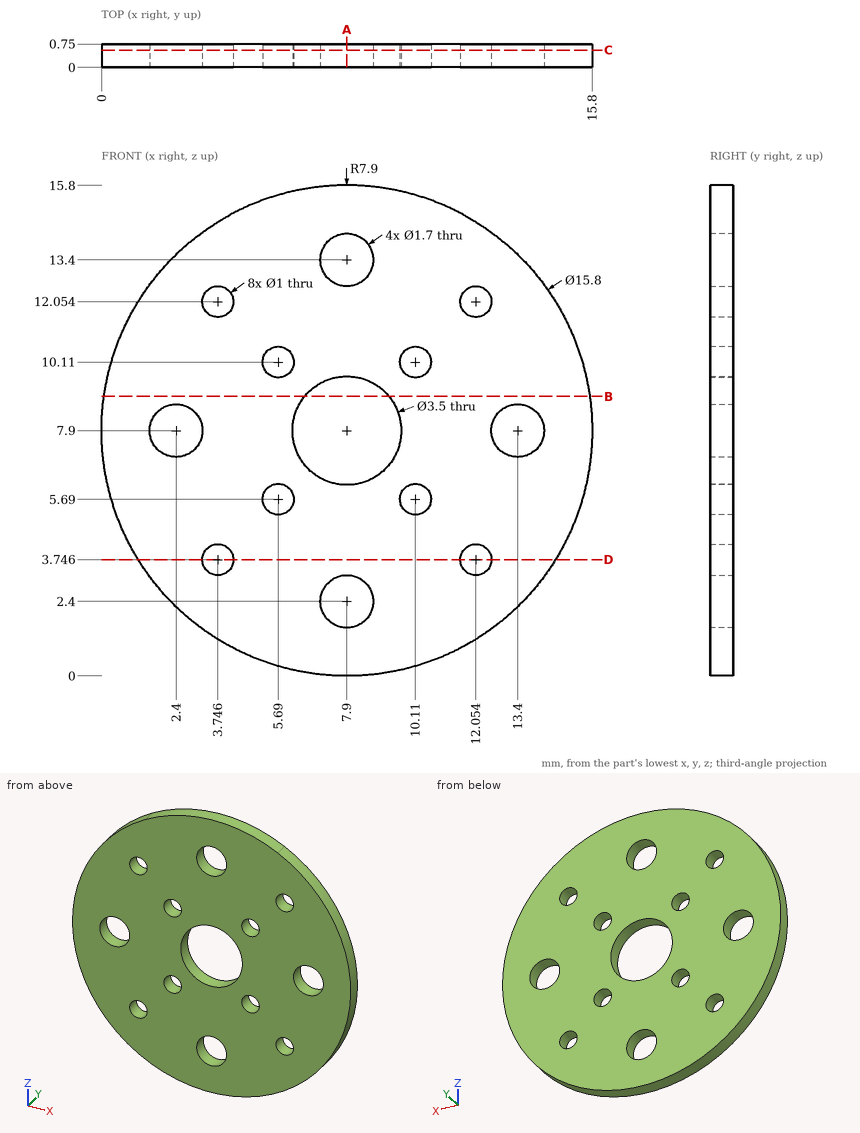
Answer from the drawing. Dimensions are ordinates in mm from the lowest x, y and z of the part. Coordinates: 2 decimals unless noted, no trailing zeros. Loops run counter-clockwise (first coordinate to the right, second up) from the corner with the lowest first, then second, coordinate; pieces in that order, holes last. Notation, with made-up numbers: (28.5, -34) - (79.5, -34) arc R13 ccw to (79.5, -10) - close; hole circle Ø3 at (47.5, 85.25). An arc over 180 degrees is marked (long way). Answer in a Markdown table with one row per item.
1. Find section D-D, the plane z = 3.75. Write down the section's boundary in (x, y).
Conclusion:
| item | result |
|---|---|
| outline | (1.18, 0) - (3.25, 0) - (3.25, 0.75) - (1.18, 0.75) - close; (4.25, 0) - (11.55, 0) - (11.55, 0.75) - (4.25, 0.75) - close; (12.55, 0) - (14.62, 0) - (14.62, 0.75) - (12.55, 0.75) - close |
2. Find section A-A, the plane x = 7.9. Write down the section's boundary in (y, z), then the cut area to 4 significant figures.
Conclusion:
| item | result |
|---|---|
| outline | (0, 0) - (0.75, 0) - (0.75, 1.55) - (0, 1.55) - close; (0, 3.25) - (0.75, 3.25) - (0.75, 6.15) - (0, 6.15) - close; (0, 9.65) - (0.75, 9.65) - (0.75, 12.55) - (0, 12.55) - close; (0, 14.25) - (0.75, 14.25) - (0.75, 15.8) - (0, 15.8) - close |
| area | 6.675 mm² |
3. Find section B-B, the plane z = 9. Write down the section's boundary in (x, y), then the cut area to 3 significant figures.
Conclusion:
| item | result |
|---|---|
| outline | (0.08, 0) - (6.54, 0) - (6.54, 0.75) - (0.08, 0.75) - close; (9.26, 0) - (15.72, 0) - (15.72, 0.75) - (9.26, 0.75) - close |
| area | 9.69 mm² |
4. Find section C-C, the plane y = 0.55. Count the separate pieces of the cut face and the enclosed holes in it, then the cut area to 3 significant figures.
Conclusion:
| item | result |
|---|---|
| separate pieces | 1 |
| enclosed holes | 13 |
| area | 171 mm² |
5. Straight lines are drawn through the part: line 1 (X direction, y = 0.65, z = 7.9); line 2 (X direction, y = 0.5, z = 4). For each, find the intervals that lie inside material, in ascending order.
Conclusion:
| item | result |
|---|---|
| line 1 | x = 0 to 1.55, 3.25 to 6.15, 9.65 to 12.55, 14.25 to 15.8 |
| line 2 | x = 1.03 to 3.32, 4.18 to 11.62, 12.48 to 14.77 |
